Source: three-view drawing plus pictorial views. Frame: mm from the lowest corner of the part. Give positions to 0.01 mm unless a question says otherwise; leave off trailing zeros. Write each loop counter-clockwise with the first axis right and the second up, starting at its lowest first coordinate (ties: lowest second). Pieces come first, ordered by that corner, then holes. Notation, with made-up numbers: (55.5, -40) -> (79.5, -40) arc R23 ccw to (79.5, -3) -> close; hole circle Ø10 at (87.25, 48). An arc over 180 degrees is marked (long way). Use a Markdown table: item, result. Add a question column.
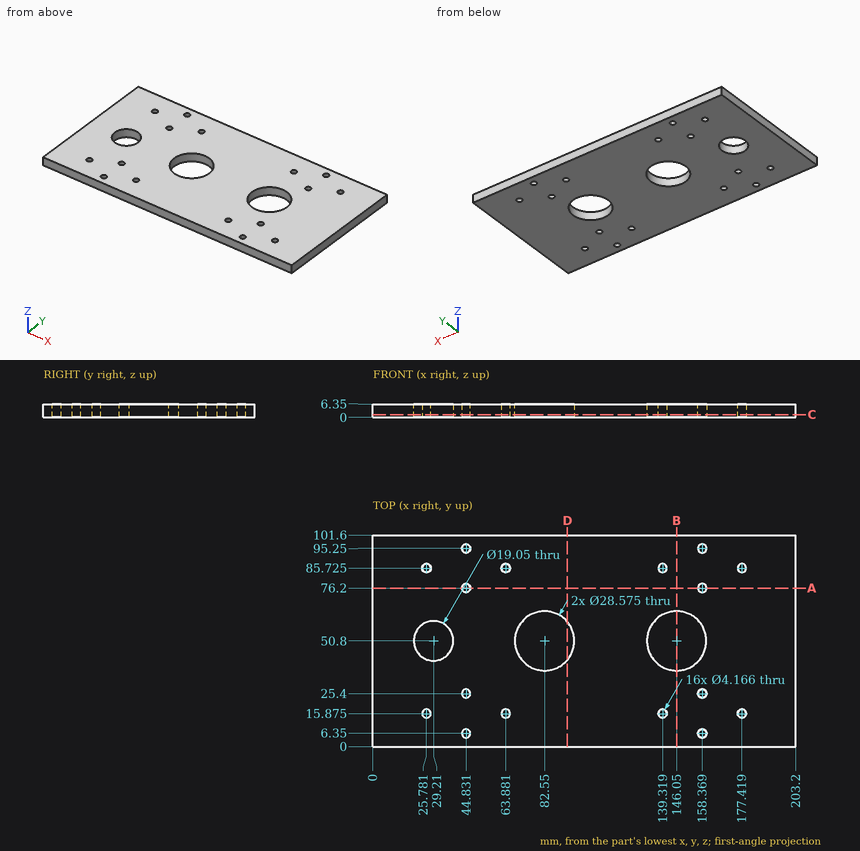
(1) Cut plane C-C on z = 1.25. Count the separate pieces of the cut face and the enclosed holes in it, then the cut area to 3 significant figures.
(2) Cut plane B-B on x = 146.05. Return the cut outline in (y, z), then the cut area to 3 significant figures.
(3) Cut plane D-D on x = 93.5. Return the cut outline in (y, z).
(4) Cut plane A-A on y = 76.2. Return the cut outline in (x, z), then the cut area to 3 significant figures.
(5) Material intervals for L1, parallel to Y at x = 177.5, z = 1.25; L2, parallel to Y at x = 178, z = 2.75 (1 decimal); L3, parallel to X at y = 7.5, z = 1.5 (1 decimal), sorted ascending.
(6) First-contact query: pin 1 Ø2.5 at (x, y) = (158.369, 6.35) entering from +Z. Flat tip, straight axial feed; report the tip coordinate or a pass-through.
Output:
| question | item | result |
|---|---|---|
| 1 | separate pieces | 1 |
| 1 | enclosed holes | 19 |
| 1 | area | 18,900 mm^2 |
| 2 | outline | (0, 0) -> (36.51, 0) -> (36.51, 6.35) -> (0, 6.35) -> close; (65.09, 0) -> (101.6, 0) -> (101.6, 6.35) -> (65.09, 6.35) -> close |
| 2 | area | 464 mm^2 |
| 3 | outline | (0, 0) -> (41.62, 0) -> (41.62, 6.35) -> (0, 6.35) -> close; (59.98, 0) -> (101.6, 0) -> (101.6, 6.35) -> (59.98, 6.35) -> close |
| 4 | outline | (0, 0) -> (42.75, 0) -> (42.75, 6.35) -> (0, 6.35) -> close; (46.91, 0) -> (156.29, 0) -> (156.29, 6.35) -> (46.91, 6.35) -> close; (160.45, 0) -> (203.2, 0) -> (203.2, 6.35) -> (160.45, 6.35) -> close |
| 4 | area | 1,240 mm^2 |
| 5 | L1 | 0 to 13.79, 17.96 to 83.64, 87.81 to 101.6 |
| 5 | L2 | 0 to 13.9, 17.9 to 83.7, 87.7 to 101.6 |
| 5 | L3 | 0 to 43.1, 46.6 to 156.6, 160.1 to 203.2 |
| 6 | pin 1 | through |
